Build history of the part. All positions in model axes, mm. Round coordinates to 2 decimals unless told otherwise and drop trailing zeros. Order: outer loops, then holes, each group sorted by start corner. A loop starts at its lowest first (then second) coordinate and runs counter-clockwise, first axis right, second up. Notation, with made-up numbers: (-4, 69.5) -> (8, 69.5) arc R10 ccw to (8, 85.5) -> close; hole circle Ø1 at (9, -2). An arc over 180 degrees is marked (long way). Write item = value, one per line.
from build123d import *

# Parameters (mm, degrees)
DOME1_FACE_RADIUS = 15
DOME1_HEIGHT      = 65
DOME2_FACE_RADIUS = 15
DOME2_HEIGHT      = 65


with BuildPart() as part:
    # Sketch2 → Revolve1 (revolve)
    with BuildSketch(Plane.XY):
        Polygon((-265, 0), (265, 0), (265, 15), (250, 15), (200, 30), (-200, 30), (-250, 15), (-265, 15), align=None)
    revolve(axis=Axis((-265, 0, 0), (1, 0, 0)))

    # Dome1: a dome of height H over a round flat face of radius A is a cap of a sphere of radius (A * A + H * H) / (2 * H)
    dome1_r = (DOME1_FACE_RADIUS * DOME1_FACE_RADIUS + DOME1_HEIGHT * DOME1_HEIGHT) / (2 * DOME1_HEIGHT)
    dome1_base = Plane((265, 0, 0), z_dir=(1, 0, 0))
    with Locations(dome1_base.offset(DOME1_HEIGHT - dome1_r)):
        dome1_ball = Sphere(dome1_r, mode=Mode.PRIVATE)
    add(split(dome1_ball, bisect_by=dome1_base, keep=Keep.TOP, mode=Mode.PRIVATE))

    # Dome2: a dome of height H over a round flat face of radius A is a cap of a sphere of radius (A * A + H * H) / (2 * H)
    dome2_r = (DOME2_FACE_RADIUS * DOME2_FACE_RADIUS + DOME2_HEIGHT * DOME2_HEIGHT) / (2 * DOME2_HEIGHT)
    dome2_base = Plane((-265, 0, 0), z_dir=(-1, 0, 0))
    with Locations(dome2_base.offset(DOME2_HEIGHT - dome2_r)):
        dome2_ball = Sphere(dome2_r, mode=Mode.PRIVATE)
    add(split(dome2_ball, bisect_by=dome2_base, keep=Keep.TOP, mode=Mode.PRIVATE))


solid = part.part
Q1. Cut at D-D, the plane y = 24. Give the number of separate pieces and of enclosed holes in the cut face, and give its area (3 significant figures).
Check values:
separate_pieces = 3
enclosed_holes = 0
area = 19,100 mm²
Q2. Flat gauge pins, fed straight in: pin 1 (12 mm diameter, centred on x = -81, y = -11, fed in from -Z); pin 2 (3 mm diameter, centred on x = -237, y = -9.5, fed in from -Z); pin 3 (8 mm diameter, centred on x = -212.5, z = 26.5, fed in from +Y). Where does each tip first touch, or does it go through?
Check values:
pin_1 = -29.58
pin_2 = -17.28
pin_3 = 13.91
Q3. Probe probe 1 along Z at (x, y) = (-247.5, -5); probe 2 along Y at (x, z) = (-189.5, -26); probe 3 along Z at (x, y) = (-99, 10). List the from-to ranges inside material, lowest first.
Check values:
probe_1 = -14.94 to 14.94
probe_2 = -14.97 to 14.97
probe_3 = -28.28 to 28.28
Q4. Cut at A-A, the plane y = 0. List the corners of the cut face in (x, z).
Check values:
outline = (-265, -15) -> (-250, -15) -> (-200, -30) -> (200, -30) -> (250, -15) -> (265, -15) arc R34.23 ccw (long way) to (265, 15) -> (250, 15) -> (200, 30) -> (-200, 30) -> (-250, 15) -> (-265, 15) arc R34.23 ccw (long way) to start
Q5. Cut at C-C, the plane x = 161. List the corners of the cut face in (y, z), and give its area (3 significant figures).
Check values:
outline = circle Ø60 at (0, 0)
area = 2,830 mm²
